from build123d import *

# Parameters (mm, degrees)
SKETCH1_R           = 6.8
SKETCH1_R_2         = 5
BOSS_EXTRUDE1_DEPTH = 1
BOSS_EXTRUDE2_DEPTH = 1
FILLET1_R           = 1
SKETCH3_W           = 1
SKETCH3_H           = 3.309988885
CUT_EXTRUDE1_DEPTH  = 11.764757313
SKETCH4_R           = 0.75
CUT_EXTRUDE2_DEPTH  = 11.764757313


with BuildPart() as part:
    # Sketch1 → Boss-Extrude1 (new body)
    with BuildSketch(Plane(origin=(0, 0, 0), x_dir=(1, 0, 0), z_dir=(0, 1, 0))):
        with Locations(Location((0, 0, 0), (0, 0, 270))):
            Circle(SKETCH1_R)
        with Locations(Location((0, 0, 0), (0, 0, 270))):
            Circle(SKETCH1_R_2, mode=Mode.SUBTRACT)
    extrude(amount=BOSS_EXTRUDE1_DEPTH)

    # Sketch2 → Boss-Extrude2 (add)
    with BuildSketch(Plane.XZ):
        with BuildLine():
            Line((3, -7.738862966), (3, -6.102458521))
            ThreePointArc((3, -6.102458521), (1.782640126, -6.562179073), (0.5, -6.781592733))
            Line((0.5, -6.781592733), (0.5, -8.284926071))
            ThreePointArc((0.5, -8.284926071), (1.771170864, -8.108819505), (3, -7.738862966))
        make_face()
        with BuildLine():
            Line((-0.5, -8.284926071), (-0.5, -6.781592733))
            ThreePointArc((-0.5, -6.781592733), (-1.782640126, -6.562179073), (-3, -6.102458521))
            Line((-3, -6.102458521), (-3, -7.738862966))
            ThreePointArc((-3, -7.738862966), (-1.771170864, -8.108819505), (-0.5, -8.284926071))
        make_face()
    extrude(amount=-BOSS_EXTRUDE2_DEPTH)

    # Fillet1
    fillet1_edges = [part.edges().sort_by_distance(p)[0] for p in [
        (3, 0.5, -7.738862966),
        (-3, 0.5, -7.738862966),
    ]]
    fillet(fillet1_edges, radius=FILLET1_R)

    # Sketch3 → Cut-Extrude1 (cut, through all)
    with BuildSketch(Plane.XZ):
        with Locations((0, -6.629931629)):
            Rectangle(SKETCH3_W, SKETCH3_H)
    extrude(amount=-CUT_EXTRUDE1_DEPTH, mode=Mode.SUBTRACT)

    # Sketch4 → Cut-Extrude2 (cut, through all)
    with BuildSketch(Plane.XZ):
        with Locations(Location((1.707693317, -6.821038057, 0), (0, 0, 270))):
            Circle(SKETCH4_R)
        with Locations(Location((-1.707693317, -6.821038057, 0), (0, 0, 90))):
            Circle(SKETCH4_R)
    extrude(amount=-CUT_EXTRUDE2_DEPTH, mode=Mode.SUBTRACT)


solid = part.part
Read the model definition and answer for the solid it produces. Units are mm, in the model's axes. A direction names the side the tool comes from. Coordinates: 2 decimals unless noted, no trailing zeros. Write each loop counter-clockwise with the first axis right and the second up, starting at its lowest first coordinate (ties: lowest second). Pieces come first, ordered by that corner, then holes. Notation, with made-up numbers: M 30,53.25 L 79,53.25 A20 ccw 79,82.25 Z; hole C 85,17.5 d3. An arc over 180 degrees is marked long. Use a Markdown table: item, result.
Q1. Straight lines are drawn through the part: L1, parallel to X at y = 0.2, z = -6.75; L2, parallel to X at y = 0.45, z = 0; L3, parallel to X at y = 0.8, z = -7. For each, find the intervals that lie inside material, in ascending order. Write a range as [from, to].
Answer block:
| item | result |
|---|---|
| L1 | x = [-3, -2.45], [-0.96, -0.5], [0.5, 0.96], [2.45, 3] |
| L2 | x = [-6.8, -5], [5, 6.8] |
| L3 | x = [-3, -2.44], [-0.98, -0.5], [0.5, 0.98], [2.44, 3] |
Q2. The part is cut by section B-B, the plane y = 0.45. Write down the section's boundary in (x, z), then the cut area to 3 significant figures.
Answer block:
| item | result |
|---|---|
| outline | M -3,-7.02 A1 ccw -2.27,-7.98 A8.3 ccw -0.5,-8.28 L -0.5,-4.97 A5 cw long 0.5,-4.97 L 0.5,-8.28 A8.3 ccw 2.27,-7.98 A1 ccw 3,-7.02 L 3,-6.1 A6.8 ccw long -3,-6.1 Z; hole C -1.71,-6.82 d1.5; hole C 1.71,-6.82 d1.5 |
| area | 68.9 mm2 |
Q3. The part is cut by section A-A, the plane z = 0. Write down the section's boundary in (x, y).
Answer block:
| item | result |
|---|---|
| outline | M -6.8,0 L -5,0 L -5,1 L -6.8,1 Z; M 5,0 L 6.8,0 L 6.8,1 L 5,1 Z |
Q4. Which of the six approach directions +Z, -Z, +X, -X, +Y, -Y give full straight-line access (tool end or side, diameter ignored) to faces 1 (the face through (3, 0.5, -6.6)), 2 (the face through (-3, 0.5, -6.6)), 3 (the face through (-0.5, 0.5, -6.7))?
Answer block:
| item | result |
|---|---|
| face 1 | -Z, +X, +Y, -Y |
| face 2 | -Z, -X, +Y, -Y |
| face 3 | -Z, +Y, -Y |
Q5. The part is cut by section C-C, the plane z = -6.5. Write down the section's boundary in (x, y).
Answer block:
| item | result |
|---|---|
| outline | M -3,0 L -2.39,0 L -2.39,1 L -3,1 Z; M -1.03,0 L -0.5,0 L -0.5,1 L -1.03,1 Z; M 0.5,0 L 1.03,0 L 1.03,1 L 0.5,1 Z; M 2.39,0 L 3,0 L 3,1 L 2.39,1 Z |
Q6. The part is cut by section D-D, the plane x = -4.25. Write down the section's boundary in (y, z).
Answer block:
| item | result |
|---|---|
| outline | M 0,-5.31 L 1,-5.31 L 1,-2.63 L 0,-2.63 Z; M 0,2.63 L 1,2.63 L 1,5.31 L 0,5.31 Z |
Q7. Each of these flat-tipped pins is pushed along its axis until it touches: pin 1 Ø0.5 at (y, z) = (0.5, -6.5) entering from +X; pin 2 Ø0.5 at (y, z) = (0.5, -6) entering from +X. Where does it stop, or does it pass through?
Answer block:
| item | result |
|---|---|
| pin 1 | stops at x = 3 |
| pin 2 | stops at x = 3.63 |
